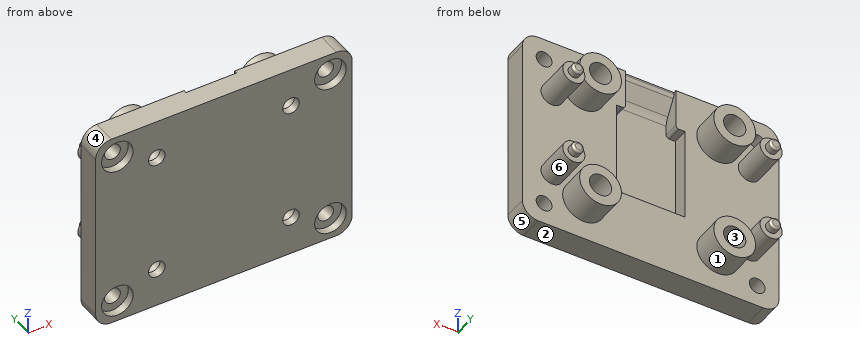
from build123d import *

# Parameters (mm, degrees)
SKETCH_1_W          = 32.5
SKETCH_1_H          = 25.5
EXTRUDE_1_DEPTH     = 3
EXTRUDE_2_DEPTH     = 1.5
SKETCH_5_R          = 1.4
EXTRUDE_3_DEPTH     = 4.5
SKETCH_6_R          = 0.725
EXTRUDE_4_DEPTH     = 1
SKETCH_7_R          = 1
CUT_EXTRUDE_1_DEPTH = 10
SKETCH_8_R          = 2
CUT_EXTRUDE_2_DEPTH = 1
FILLET_1_R          = 2
SKETCH_9_R          = 2.65
EXTRUDE_5_DEPTH     = 3.5
SKETCH_11_R         = 1.05
CUT_EXTRUDE_4_DEPTH = 100
SKETCH_12_R         = 1.41
CUT_EXTRUDE_5_DEPTH = 5.5
FILLET_2_R          = 0.3
CUT_EXTRUDE_8_DEPTH = 2
CUT_EXTRUDE_9_DEPTH = 1.5
EXTRUDE_6_DEPTH     = 6.4
FILLET_3_R          = 2
FILLET_5_R          = 1
FILLET_6_R          = 0.4


with BuildPart() as part:
    # 草图1 → 凸台-拉伸1 (new body)
    with BuildSketch(Plane(origin=(0, 0, 0), x_dir=(1, 0, 0), z_dir=(0, 1, 0))):
        Rectangle(SKETCH_1_W, SKETCH_1_H)
    extrude(amount=EXTRUDE_1_DEPTH)

    # 草图2 → 凸台-拉伸2 (add)
    with BuildSketch(Plane(origin=(0, 3, 0), x_dir=(1, 0, 0), z_dir=(0, 1, 0))):
        Polygon((-5.35, 5.35), (5.35, 5.35), (5.35, -7.55), (4.35, -7.55), (4.35, 4.35), (-4.35, 4.35), (-4.35, -7.55), (-5.35, -7.55), align=None)
    extrude(amount=EXTRUDE_2_DEPTH)

    # 草图5 → 凸台-拉伸3 (add)
    with BuildSketch(Plane(origin=(0, 3, 0), x_dir=(1, 0, 0), z_dir=(0, 1, 0))):
        with Locations((12.5, 5.5)):
            Circle(SKETCH_5_R)
        with Locations((12.5, -5.5)):
            Circle(SKETCH_5_R)
        with Locations((-12.5, -5.5)):
            Circle(SKETCH_5_R)
        with Locations((-12.5, 5.5)):
            Circle(SKETCH_5_R)
    extrude(amount=EXTRUDE_3_DEPTH)

    # 草图6 → 凸台-拉伸4 (add)
    with BuildSketch(Plane(origin=(0, 7.5, 0), x_dir=(1, 0, 0), z_dir=(0, 1, 0))):
        with Locations((-12.5, -5.5)):
            Circle(SKETCH_6_R)
        with Locations((-12.5, 5.5)):
            Circle(SKETCH_6_R)
        with Locations((12.5, 5.5)):
            Circle(SKETCH_6_R)
        with Locations((12.5, -5.5)):
            Circle(SKETCH_6_R)
    extrude(amount=EXTRUDE_4_DEPTH)

    # 草图7 → 切除-拉伸1 (cut)
    with BuildSketch(Plane(origin=(0, 3, 0), x_dir=(1, 0, 0), z_dir=(0, 1, 0))):
        with Locations((13.5, 10)):
            Circle(SKETCH_7_R)
        with Locations((-13.5, 10)):
            Circle(SKETCH_7_R)
        with Locations((-13.5, -10)):
            Circle(SKETCH_7_R)
        with Locations((13.5, -10)):
            Circle(SKETCH_7_R)
    extrude(amount=-CUT_EXTRUDE_1_DEPTH, mode=Mode.SUBTRACT)

    # 草图8 → 切除-拉伸2 (cut)
    with BuildSketch(Plane.XZ):
        with Locations((-13.5, 10)):
            Circle(SKETCH_8_R)
        with Locations((13.5, 10)):
            Circle(SKETCH_8_R)
        with Locations((13.5, -10)):
            Circle(SKETCH_8_R)
        with Locations((-13.5, -10)):
            Circle(SKETCH_8_R)
    extrude(amount=-CUT_EXTRUDE_2_DEPTH, mode=Mode.SUBTRACT)

    # 圆角1
    fillet_1_edges = [part.edges().sort_by_distance(p)[0] for p in [
        (16.25, 1.5, 12.75),
        (-16.25, 1.5, 12.75),
        (-16.25, 1.5, -12.75),
        (16.25, 1.5, -12.75),
    ]]
    fillet(fillet_1_edges, radius=FILLET_1_R)

    # 草图9 → 凸台-拉伸5 (add)
    with BuildSketch(Plane(origin=(0, 3, 0), x_dir=(1, 0, 0), z_dir=(0, 1, 0))):
        with Locations((8.5, 7.75)):
            Circle(SKETCH_9_R)
        with Locations((-8.5, 7.75)):
            Circle(SKETCH_9_R)
        with Locations((-8.5, -7.75)):
            Circle(SKETCH_9_R)
        with Locations((8.5, -7.75)):
            Circle(SKETCH_9_R)
    extrude(amount=EXTRUDE_5_DEPTH)

    # 草图11 → 切除-拉伸4 (cut)
    with BuildSketch(Plane(origin=(0, 6.5, 0), x_dir=(1, 0, 0), z_dir=(0, 1, 0))):
        with Locations((-8.5, 7.75)):
            Circle(SKETCH_11_R)
        with Locations((-8.5, -7.75)):
            Circle(SKETCH_11_R)
        with Locations((8.5, -7.75)):
            Circle(SKETCH_11_R)
        with Locations((8.5, 7.75)):
            Circle(SKETCH_11_R)
    extrude(amount=-CUT_EXTRUDE_4_DEPTH, mode=Mode.SUBTRACT)

    # 草图12 → 切除-拉伸5 (cut)
    with BuildSketch(Plane(origin=(0, 6.5, 0), x_dir=(1, 0, 0), z_dir=(0, 1, 0))):
        with Locations((-8.5, 7.75)):
            Circle(SKETCH_12_R)
        with Locations((8.5, 7.75)):
            Circle(SKETCH_12_R)
        with Locations((-8.5, -7.75)):
            Circle(SKETCH_12_R)
        with Locations((8.5, -7.75)):
            Circle(SKETCH_12_R)
    extrude(amount=-CUT_EXTRUDE_5_DEPTH, mode=Mode.SUBTRACT)

    # 圆角2
    fillet_2_edges = [part.edges().sort_by_distance(p)[0] for p in [
        (-13.225, 8.5, 5.5),
        (-13.225, 8.5, -5.5),
        (11.775, 8.5, -5.5),
        (11.775, 8.5, 5.5),
    ]]
    fillet(fillet_2_edges, radius=FILLET_2_R)

    # 草图15 → 切除-拉伸8 (cut)
    with BuildSketch(Plane(origin=(0, 3, 0), x_dir=(1, 0, 0), z_dir=(0, 1, 0))):
        Polygon((-4.35, 4.35), (4.35, 4.35), (4.35, -7.55), (3.2, -7.55), (3.2, -12.75), (-3.2, -12.75), (-3.2, -7.55), (-4.35, -7.55), align=None)
    extrude(amount=-CUT_EXTRUDE_8_DEPTH, mode=Mode.SUBTRACT)

    # 草图17 → 切除-拉伸9 (cut)
    with BuildSketch(Plane(origin=(0, 4.5, 0), x_dir=(1, 0, 0), z_dir=(0, 1, 0))):
        Polygon((-4.35, -7.55), (-4.35, 4.35), (4.35, 4.35), (4.35, -7.55), (5.35, -7.55), (5.35, 5.35), (-5.35, 5.35), (-5.35, -7.55), align=None)
    extrude(amount=-CUT_EXTRUDE_9_DEPTH, mode=Mode.SUBTRACT)

    # 草图18 → 凸台-拉伸6 (add)
    with BuildSketch(Plane.ZY.offset(-3.2)):
        Polygon((12.75, 1), (9.75, 1), (12.25, 2.6), (12.75, 2.6), align=None)
    extrude(amount=EXTRUDE_6_DEPTH)

    # 圆角3
    fillet_3_edges = [part.edges().sort_by_distance(p)[0] for p in [
        (0, 1, 9.75),
    ]]
    fillet(fillet_3_edges, radius=FILLET_3_R)

    # 圆角5
    fillet_5_edges = [part.edges().sort_by_distance(p)[0] for p in [
        (0, 2.6, 12.25),
    ]]
    fillet(fillet_5_edges, radius=FILLET_5_R)

    # 圆角6
    fillet_6_edges = [part.edges().sort_by_distance(p)[0] for p in [
        (3.2, 2, 7.55),
        (-3.2, 2, 7.55),
    ]]
    fillet(fillet_6_edges, radius=FILLET_6_R)


solid = part.part
The listing builds one solid part. Answer for the finished solid, in the listing's coordinates (mm). Face numbers are marked on the shaded views. A direction names the side the tool comes from. Give positions to 0.01 mm unless a question says otherwise; leave off trailing zeros. Write each loop counter-clockwise with the first axis right and the second up, starting at its lowest first coordinate (ties: lowest second). Pieces come first, ordered by that corner, then holes.
1) Section C-C (x = -8.5) is taken. Write down the section's boundary in (y, z).
2) Section B-B (z = -10) is taken. Write down the section's boundary in (x, y), and give its area (3 significant figures).
3) Given P1, Ø2, axis at x = -13, z = -9.5, coming from the -Y side; P2, Ø5, axis at x = 6, y = 7, coming from the +Z side; P3, Ø1.5, axis at x = -9, z = -8.5, coming from the +Y side; P4, Ø1.7, axis at x = -8.5, z = 7.75, coming from the +Y side, each flat-ended and moving along its own axis, determine where each tip first touches the part or whether it passes through.
4) A tool of negligible diameter and unlimited length cuts with its end or side. For the marked faces 5 and 6, from which of +Z, -Z, +X, -X, +Y, -Y can it reach the whole face along a straight path? Write none if from no direction.
5) For a pull along X with two mould halves and no side action, classify the marked faces 1, 2, 3 and 4 as pulls with the +X half, pulls with the -X half, needs draft (parallel to the pull), parting line crosses it, or undercut.
6) Find the intervals of material crossed by L1, parallel to X at y = 0.55, z = -7.75; L2, parallel to Z at x = 13.5, y = 1.55; L3, parallel to Z at x = -8.5, y = 3.95, in increasing order.
7) Section D-D (x = 2) is taken. Write down the section's boundary in (y, z).
8) Section A-A (y = 5.25) is taken. Count the separate pieces of the cut face and the enclosed holes in it, and give its area (3 significant figures).
Response:
1. outline: (0, -12.75) - (3, -12.75) - (3, -10.4) - (6.5, -10.4) - (6.5, -9.16) - (1, -9.16) - (1, -8.8) - (0, -8.8) - close; (0, -6.7) - (1, -6.7) - (1, -6.34) - (6.5, -6.34) - (6.5, -5.1) - (3, -5.1) - (3, 5.1) - (6.5, 5.1) - (6.5, 6.34) - (1, 6.34) - (1, 6.7) - (0, 6.7) - close; (0, 8.8) - (1, 8.8) - (1, 9.16) - (6.5, 9.16) - (6.5, 10.4) - (3, 10.4) - (3, 12.75) - (0, 12.75) - close
2. outline: (-16.25, 0) - (-15.5, 0) - (-15.5, 1) - (-14.5, 1) - (-14.5, 3) - (-16.25, 3) - close; (-12.5, 1) - (-11.5, 1) - (-11.5, 0) - (11.5, 0) - (11.5, 1) - (12.5, 1) - (12.5, 3) - (9.9, 3) - (9.9, 6.5) - (7.1, 6.5) - (7.1, 3) - (-7.1, 3) - (-7.1, 6.5) - (-9.9, 6.5) - (-9.9, 3) - (-12.5, 3) - close; (14.5, 1) - (15.5, 1) - (15.5, 0) - (16.25, 0) - (16.25, 3) - (14.5, 3) - close
2. area: 101 mm2
3. P1: stops at y = 1
3. P2: stops at z = 10.4
3. P3: stops at y = 6.5
3. P4: passes through
4. face 5: -Z, +X, +Y, -Y
4. face 6: +Y
5. face 1: undercut
5. face 2: needs draft
5. face 3: undercut
5. face 4: pulls with the -X half
6. L1: x = -16.25 to -9.55, -7.45 to 7.45, 9.55 to 16.25
6. L2: z = -12.75 to -11, -9 to 9, 11 to 12.75
6. L3: z = -10.4 to -9.16, -6.34 to -5.1, 5.1 to 6.34, 9.16 to 10.4
7. outline: (0, -12.75) - (3, -12.75) - (3, -4.35) - (1, -4.35) - (1, 9.16) arc R2 cw to (1.32, 10.24) - (2.44, 12) arc R1 ccw to (2.6, 12.54) - (2.6, 12.75) - (0, 12.75) - close
8. separate pieces: 8
8. enclosed holes: 4
8. area: 87.9 mm2
